from build123d import *

# Parameters (mm, degrees)
F0_R     = 0.8
F1_DEPTH = 2


with BuildPart() as f1:
    # F0 (on Top) → F1 (new body)
    with BuildSketch(Plane.XY):
        with BuildLine():
            ThreePointArc((2, 3), (1.4142135624, 4.4142135624), (0, 5))
            ThreePointArc((0, 5), (-1.4142135624, 4.4142135624), (-2, 3))
            ThreePointArc((-2, 3), (0, 1), (2, 3))
        make_face()
        with Locations((0, 3)):
            Circle(F0_R, mode=Mode.SUBTRACT)
        with BuildLine():
            ThreePointArc((2, 3), (0, 1), (-2, 3))
            Line((-2, 3), (-2, -3))
            ThreePointArc((-2, -3), (0, -1), (2, -3))
            Line((2, -3), (2, 3))
        make_face()
        with BuildLine():
            ThreePointArc((2, -3), (0, -1), (-2, -3))
            ThreePointArc((-2, -3), (-1.4142135624, -4.4142135624), (0, -5))
            ThreePointArc((0, -5), (1.4142135624, -4.4142135624), (2, -3))
        make_face()
        with Locations((0, -3)):
            Circle(F0_R, mode=Mode.SUBTRACT)
    extrude(amount=F1_DEPTH)


solid = f1.part
Input: part model. Units: mm. Frame: model coordinates. Coordinates: 2 decimals unless noted, no trailing zeros. Loops run counter-clockwise (first coordinate to the right, second up) from the corner with the lowest first, then second, coordinate; pieces in that order, holes last. Notation, with made-up numbers: (-31.5, -32) -> (-23.5, -32) arc R17 ccw to (-23.5, 0) -> close; hole circle Ø4 at (38.5, 6). An arc over 180 degrees is marked (long way). Write each question's results on one line, items separated by ' | '. Start each with the question number.
Q1. Section B-B, the plane x = 0.45. Return the cut outline in (y, z), plus the area to 3 significant figures.
Q2. Section C-C, the plane y = -4.5. Return the cut outline in (x, z).
Q3. Ray query, line 1 (Y direction, x = 0.3, z = 1); line 2 (Y direction, x = -0.6, z = 1.15); line 3 (X direction, y = -4.25, z = 0.6). Return the intervals inside material, ascending. Write a range as from..to.
Q4. Pull-direction query (Y, two-part tool) for faces 1 (the flat face through (-2, 0, 1)), 2 (the cylindrical face through (-0.17, -3.78, 0.99)); classes: released by +Y, released by -Y, zero draft, split by the parting line, or undercut.
Q5. Pin query (flat end, axial travel): pin 1 (1 mm diameter, centred on x = 0, y = 3, fed in from +Z); pin 2 (1 mm diameter, centred on x = 1, z = 1.5, fed in from +Y). Return the tip coordinate at first contact, or that it passes through.
Q6. Section A-A, the plane z = 0.7. Return the cut outline in (x, y), plus the area to 3 significant figures.
Q7. Section D-D, the plane x = -0.3. Return the cut outline in (y, z), plus the area to 3 significant figures.
Found:
1) outline: (-4.95, 0) -> (-3.66, 0) -> (-3.66, 2) -> (-4.95, 2) -> close; (-2.34, 0) -> (2.34, 0) -> (2.34, 2) -> (-2.34, 2) -> close; (3.66, 0) -> (4.95, 0) -> (4.95, 2) -> (3.66, 2) -> close | area: 14.5 mm2
2) outline: (-1.32, 0) -> (1.32, 0) -> (1.32, 2) -> (-1.32, 2) -> close
3) line 1: -4.98..-3.74, -2.26..2.26, 3.74..4.98 | line 2: -4.91..-3.53, -2.47..2.47, 3.53..4.91 | line 3: -1.56..1.56
4) face 1: zero draft | face 2: undercut
5) pin 1: through | pin 2: y = 4.94
6) outline: (-2, -3) arc R2 ccw to (2, -3) -> (2, 3) arc R2 ccw to (-2, 3) -> close; hole circle Ø1.6 at (0, -3); hole circle Ø1.6 at (0, 3) | area: 32.5 mm2
7) outline: (-4.98, 0) -> (-3.74, 0) -> (-3.74, 2) -> (-4.98, 2) -> close; (-2.26, 0) -> (2.26, 0) -> (2.26, 2) -> (-2.26, 2) -> close; (3.74, 0) -> (4.98, 0) -> (4.98, 2) -> (3.74, 2) -> close | area: 14.0 mm2
